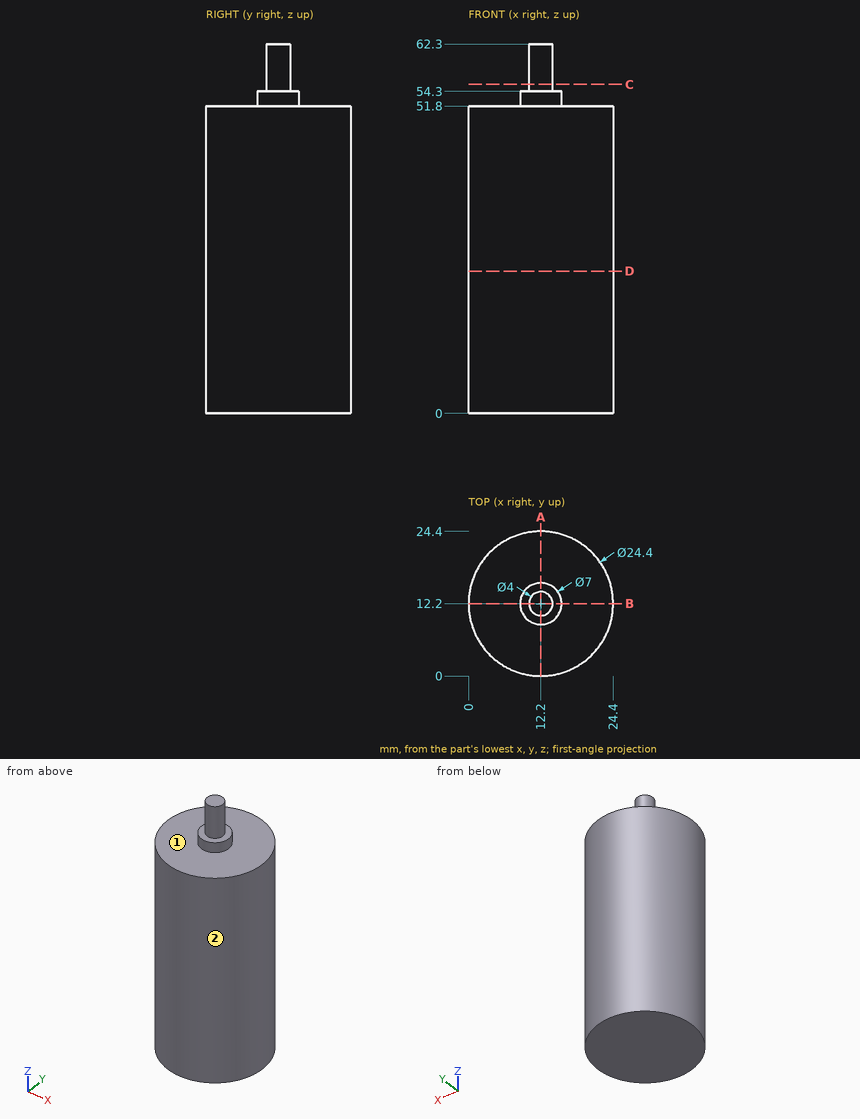
Can you work these out from the drawing? Everything is in mm from the part's minimum corner. A direction names the side the tool comes from. Coordinates: 2 decimals unless noted, no trailing zeros. Write each loop counter-clockwise with the first axis right and the second up, starting at its lowest first coordinate (ties: lowest second). Pieces come first, ordered by that corner, then holes. Notation, with made-up numbers: (-6.75, 40.5) -> (8.25, 40.5) arc R13 ccw to (8.25, 51.5) -> close; hole circle Ø5 at (86.5, 49). An arc over 180 degrees is marked (long way). Return JSON: item names as keys, results as strings.
(1) Imagine slicing it at D-D, the plane z = 24. Please give me the cut outline in (x, y), then the cut area to 3 significant figures.
Numbers:
{"outline": "circle Ø24.4 at (12.2, 12.2)", "area": "468 mm2"}
(2) Imagine slicing it at C-C, the plane z = 55.5. Please give me the cut outline in (x, y), then the cut area to 3 significant figures.
Numbers:
{"outline": "circle Ø4 at (12.2, 12.2)", "area": "12.6 mm2"}
(3) I'm going to push flat-ended pins straight in: pin 1 (2 mm diameter, centred on x = 9.5, z = 21, fed in from +Y); pin 2 (2 mm diameter, centred on y = 19, z = 50.5, fed in from +X); pin 3 (8 mm diameter, centred on y = 4, z = 8.5, fed in from +X). Where does each tip first touch, or does it pass through?
Numbers:
{"pin 1": "stops at y = 24.28", "pin 2": "stops at x = 22.93", "pin 3": "stops at x = 23.65"}
(4) Imagine slicing it at A-A, the plane x = 12.2. Please give me the cut outline in (y, z).
Numbers:
{"outline": "(0, 0) -> (24.4, 0) -> (24.4, 51.8) -> (15.7, 51.8) -> (15.7, 54.3) -> (14.2, 54.3) -> (14.2, 62.3) -> (10.2, 62.3) -> (10.2, 54.3) -> (8.7, 54.3) -> (8.7, 51.8) -> (0, 51.8) -> close"}
(5) I need wall thicknesses on L1, parallel to Z at x = 4.75, y = 6; L2, parallel to Z at x = 9.5, y = 13; L3, parallel to Y at x = 11, z = 13. Which ranges of each line are inside material? Lowest first, please.
Numbers:
{"L1": "z = 0 to 51.8", "L2": "z = 0 to 54.3", "L3": "y = 0.06 to 24.34"}
(6) Which directions (+Z, -Z, +X, -X, +Y, -Y) give clear straight access to the entire face, cutting with the end or side of a thin tool? Please do the marked faces 1 and 2.
Numbers:
{"face 1": "+Z", "face 2": "+Z, -Z"}
